Build history of the part. All positions in model axes, mm. A direction names the side the tool comes from. Round coordinates to 2 decimals unless told otherwise and drop trailing zeros. Loops run counter-clockwise (first coordinate to the right, second up) from the corner with the lowest first, then second, coordinate; pieces in that order, holes last. Notation, with made-up numbers: M 0.5,-17 L 56.5,-17 A28 cw 56.5,5 Z; hole C 45.25,85 d7. An arc over 180 degrees is marked long. Write each question's results on one line, items separated by ' | '. Start each with the question number.
```python
from build123d import *

# Parameters (mm, degrees)
EXTRUDE_1_DEPTH          = 3
SKETCH_2_OUTSIDE_W       = 13.724
SKETCH_2_OUTSIDE_H       = 8.024
CUT_EXTRUDE_1_DEPTH      = 12
SKETCH_3_R               = 1.05
CUT_EXTRUDE_2_DEPTH      = 12
SKETCH_4_R               = 0.95
EXTRUDE_2_DEPTH          = 4
SKETCH_5_W               = 12
SKETCH_5_H               = 3
EXTRUDE_3_DEPTH          = 8
SKETCH_6_R               = 1.05
CUT_EXTRUDE_3_DEPTH      = 12
SKETCH_8_W               = 8
SKETCH_8_H               = 4
CUT_EXTRUDE_4_DEPTH      = 8
EXTRUDE_5_DEPTH          = 2
SKETCH_12_W              = 11.6
SKETCH_12_H              = 3
EXTRUDE_8_DEPTH          = 4
FILLET_1_R               = 1
SKETCH_13_W              = 8
SKETCH_13_H              = 4
CUT_EXTRUDE_5_DEPTH      = 10
FILLET_2_R               = 1
CUT_EXTRUDE_6_DEPTH      = 21.322401433
CUT_EXTRUDE_6_DEPTH_BACK = 21.322401433
SKETCH_11_R              = 1.05


with BuildPart() as part:
    # 草图1 → 凸台-拉伸1 (new body)
    with BuildSketch(Plane(origin=(0, 0, 0), x_dir=(1, 0, 0), z_dir=(0, 1, 0))):
        Polygon((-6, 0), (6, 0), (6, -8.7), (4, -8.7), (4, -3), (-4, -3), (-4, -8.7), (-6, -8.7), align=None)
    extrude(amount=EXTRUDE_1_DEPTH)

    # 草图2 outside → 切除-拉伸1 (cut)
    with BuildSketch(Plane.ZY.offset(6)):
        with Locations((4.35, 1.5)):
            Rectangle(SKETCH_2_OUTSIDE_W, SKETCH_2_OUTSIDE_H)
        with BuildLine():
            Line((6.2, 3), (0, 3))
            Line((0, 3), (0, 0))
            Line((0, 0), (6.2, 0))
            ThreePointArc((6.2, 0), (7.7, 1.5), (6.2, 3))
        make_face(mode=Mode.SUBTRACT)
    extrude(amount=-CUT_EXTRUDE_1_DEPTH, mode=Mode.SUBTRACT)

    # 草图3 → 切除-拉伸2 (cut)
    with BuildSketch(Plane.ZY.offset(6)):
        with Locations((5.2, 1.5)):
            Circle(SKETCH_3_R)
    extrude(amount=-CUT_EXTRUDE_2_DEPTH, mode=Mode.SUBTRACT)

    # 草图4 → 凸台-拉伸2 (add)
    with BuildSketch(Plane(origin=(0, 0, 0), x_dir=(-1, 0, 0), z_dir=(0, 0, -1))):
        with Locations((0, 1.5)):
            Circle(SKETCH_4_R)
    extrude(amount=EXTRUDE_2_DEPTH)

    # 草图5 → 凸台-拉伸3 (add)
    with BuildSketch(Plane(origin=(0, 0, -4), x_dir=(-1, 0, 0), z_dir=(0, 0, -1))):
        with Locations((0, 1.5)):
            Rectangle(SKETCH_5_W, SKETCH_5_H)
    extrude(amount=EXTRUDE_3_DEPTH)

    # 草图6 → 切除-拉伸3 (cut)
    with BuildSketch(Plane(origin=(6, 0, 0), x_dir=(0, 0, -1), z_dir=(1, 0, 0))):
        with Locations(Location((10, 1.5, 0), (0, 0, 90))):
            Circle(SKETCH_6_R)
    extrude(amount=-CUT_EXTRUDE_3_DEPTH, mode=Mode.SUBTRACT)

    # 草图8 → 切除-拉伸4 (cut)
    with BuildSketch(Plane(origin=(0, 3, 0), x_dir=(1, 0, 0), z_dir=(0, 1, 0))):
        with Locations((0, 10)):
            Rectangle(SKETCH_8_W, SKETCH_8_H)
    extrude(amount=-CUT_EXTRUDE_4_DEPTH, mode=Mode.SUBTRACT)

    # 草图10 → 凸台-拉伸5 (add)
    with BuildSketch(Plane.ZY.offset(6)):
        with BuildLine():
            Line((-12, 3), (-8, 3))
            Line((-8, 3), (-8, 11))
            ThreePointArc((-8, 11), (-10, 13), (-12, 11))
            Line((-12, 11), (-12, 3))
        make_face()
    extrude_5 = extrude(amount=-EXTRUDE_5_DEPTH)

    # 镜向1: 凸台-拉伸5 across plane
    add(extrude_5.mirror(Plane(origin=(0, 0, 0), x_dir=(0, 0, 1), z_dir=(1, 0, 0))))

    # 草图12 → 凸台-拉伸8 (add)
    with BuildSketch(Plane.XY.offset(-4)):
        with Locations((0, 1.5)):
            Rectangle(SKETCH_12_W, SKETCH_12_H)
    extrude(amount=EXTRUDE_8_DEPTH)

    # 圆角1
    # the kernel refuses this fillet: 1 mm, written as the material it takes off along each edge
    with BuildSketch(Plane(origin=(6, -1.5, 0), x_dir=(-1, 0, 0), z_dir=(0, 1, 0))) as fillet_1_piece_1:
        with BuildLine():
            CenterArc((1, 0.6), FILLET_1_R, 180, 36.869897646)
            Line((0, 0.6), (-0.02, 0.6))
            Line((-0.02, 0.6), (-0.02, 0))
            Line((-0.02, 0), (0, -0.02))
            ThreePointArc((0, -0.02), (0.1, -0.02), (0.184, -0.012))
            Line((0.184, -0.012), (0.2, 0))
        make_face()
    extrude(amount=6, mode=Mode.SUBTRACT)
    with BuildSketch(Plane(origin=(-6, -1.5, 0), x_dir=(1, 0, 0), z_dir=(0, 1, 0))) as fillet_1_piece_2:
        with BuildLine():
            CenterArc((1, -0.6), FILLET_1_R, 143.130102354, 36.869897646)
            Line((0, -0.6), (-0.02, -0.6))
            Line((-0.02, -0.6), (-0.02, 0))
            Line((-0.02, 0), (0, 0.02))
            ThreePointArc((0, 0.02), (0.1, 0.02), (0.184, 0.012))
            Line((0.184, 0.012), (0.2, 0))
        make_face()
    extrude(amount=6, mode=Mode.SUBTRACT)

    # 草图13 → 切除-拉伸5 (cut)
    with BuildSketch(Plane(origin=(0, 3, 0), x_dir=(1, 0, 0), z_dir=(0, 1, 0))):
        with Locations((0, 6)):
            Rectangle(SKETCH_13_W, SKETCH_13_H)
    extrude(amount=-CUT_EXTRUDE_5_DEPTH, mode=Mode.SUBTRACT)

    # 圆角2
    # the kernel refuses this fillet: 1 mm, written as the material it takes off along each edge
    with BuildSketch(Plane(origin=(-6, 4.5, -4), x_dir=(0, 0, -1), z_dir=(0, -1, 0)), Plane(origin=(6, -1.5, -4), x_dir=(0, 0, -1), z_dir=(0, 1, 0))) as fillet_2_piece_1:
        with BuildLine():
            CenterArc((0.6, 1), FILLET_2_R, 233.130102354, 36.869897646)
            Line((0, 0.2), (-0.012, 0.184))
            ThreePointArc((-0.012, 0.184), (-0.02, 0.1), (-0.02, 0))
            Line((-0.02, 0), (0, -0.02))
            Line((0, -0.02), (0.6, -0.02))
            Line((0.6, -0.02), (0.6, 0))
        make_face()
    extrude(amount=6, mode=Mode.SUBTRACT)

    # 草图11 → 切除-拉伸6 (cut, two sides: drawn at the far end of the back side and taken through both)
    with BuildSketch(Plane.ZY.offset(4).offset(-CUT_EXTRUDE_6_DEPTH_BACK)):
        with Locations((-10, 11)):
            Circle(SKETCH_11_R)
    extrude(amount=CUT_EXTRUDE_6_DEPTH + CUT_EXTRUDE_6_DEPTH_BACK, mode=Mode.SUBTRACT)


solid = part.part
```
Item 1: Mould opens along Z. For faces 1 (the flat face through (-5.8, 1, -2)), 2 (the flat face through (-6, 5, -9)), 3 (the flat face through (0, 2, -4)) say: released by +Z, released by -Z, zero draft, split by the parting line, or undercut.
Item 2: Tool access for faces 4 (the flat face through (4, 5, -9)), 5 (the flat face through (5, 7, -8)), 6 (the cylindrical face through (-4.99, 2.06, -9.11)), 7 (the flat face through (0, 1, 3)), 8 (the flat face through (0, 0, -3)): list every direction of +Z, -Z, +X, -X, +Y, -Y with a clear straight run to the whole face (end or side of a thin tool).
Item 3: Drop flat-ended pins along their axis: pin 1 (6 mm diameter, centred on x = -3.5, y = 10, fed in from +Z); pin 2 (0.9 mm diameter, centred on y = 1.5, z = -1.5, fed in from -X); pin 3 (3.5 mm diameter, centred on x = -1.5, y = 1.5, fed in from -Z); pin 4 (2.5 mm diameter, centred on y = 1.5, z = -10, fed in from +X). Give the stop position or say it passes through.
Item 4: Saw through at A-A, the plane z = 5.2. Give the cut face in (x, y).
Item 5: Saw through at B-B, the plane y = 9. Give the cut face in (x, z), then the cut area to 3 significant figures.
Item 6: Saw through at C-C, the plane z = -10. Give the cut face in (x, y).
Item 7: Saw through at D-D, the plane x = -4.5. Give the cut face in (y, z).
Item 8: Drill centre lines: line 1 along Y through (x, z) = (4.95, 5.2); line 2 along X through (y, z) = (1.25, -8); line 3 along Y through (x, z) = (4.75, -3). Where is each one in solid material? Low to high. Write a range as [from, to].
Working result:
1) face 1: undercut | face 2: zero draft | face 3: released by -Z
2) face 4: -Z, +Y, -Y | face 5: +Z, +X, -X, +Y | face 6: +X, -X | face 7: +Z, +Y, -Y | face 8: +Z, -Z, +X, -X, -Y
3) pin 1: stops at z = -8 | pin 2: stops at x = -5.8 | pin 3: stops at z = -4 | pin 4: stops at x = 6
4) outline: M -6,0 L -4,0 L -4,0.45 L -6,0.45 Z; M -6,2.55 L -4,2.55 L -4,3 L -6,3 Z; M 4,0 L 6,0 L 6,0.45 L 4,0.45 Z; M 4,2.55 L 6,2.55 L 6,3 L 4,3 Z
5) outline: M -6,-12 L -4,-12 L -4,-8 L -6,-8 Z; M 4,-12 L 6,-12 L 6,-8 L 4,-8 Z | area: 16.0 mm²
6) outline: M -6,0 L -4,0 L -4,0.45 L -6,0.45 Z; M -6,2.55 L -4,2.55 L -4,9.95 L -6,9.95 Z; M -6,12.05 L -4,12.05 L -4,13 L -6,13 Z; M 4,0 L 6,0 L 6,0.45 L 4,0.45 Z; M 4,2.55 L 6,2.55 L 6,9.95 L 4,9.95 Z; M 4,12.05 L 6,12.05 L 6,13 L 4,13 Z
7) outline: M 0,-12 L 11,-12 A2 ccw 11,-8 L 3,-8 L 3,6.2 A1.5 ccw 0,6.2 Z; hole C 1.5,-10 d2.1; hole C 1.5,5.2 d2.1; hole C 11,-10 d2.1
8) line 1: y = [0, 0.45], [2.55, 3] | line 2: x = [-6, -4], [4, 6] | line 3: y = [0, 3]
